Build history of the part. All positions in model axes, mm. A direction names the side the tool comes from. Round coordinates to 2 decimals unless told otherwise and drop trailing zeros. Write each loop counter-clockwise with the first axis right and the second up, starting at its lowest first coordinate (ties: lowest second). Pieces come first, ordered by that corner, then holes.
Item 1: Drop flat-ended pins along their axis: pin 1 Ø4 at (y, z) = (-15, 22.5) entering from +X; pin 2 Ø5 at (y, z) = (-10.5, 54.5) entering from +X; pin 3 Ø2 at (x, y) = (33, -47) entering from -Z. Give the stop position or say it passes through.
Item 2: Band-saw the part on D-D, the plane z = 53. Write the cut outline in (x, y), then the cut area to 3 significant figures.
Item 3: Wall check: probe 1 along Y at (x, z) = (15, 14.5); probe 2 along X at (y, z) = (-12.5, 56); probe 3 along X at (y, z) = (33, 22). Give the ranges that are in metal, low to high.
Item 4: Mould opens along Y. For faces 1 (the flat face through (0, 75, 0)), 2 (the flat face through (-53, 1, 97)), 3 (the flat face through (-18, 77, 38)) say: +Y half, -Y half, draft (parallel to the pull), parting line (faces both ways), or undercut.
Item 5: 3-axis set-ups, long thin cutter, end or side, ignore diameter. For faces 4 (the flat face through (19.75, -1.04, 49.18)), 5 (the flat face through (22.52, -1.08, 50.7)): which of +Z, -Z, +X, -X, +Y, -Y reach the whole face in a straight line?
Item 6: Band-saw the part on C-C, the plane x = -63.5. Write the cut outline in (y, z).
Item 7: Band-saw the part on B-B, the plane y = -11. Write the cut outline in (x, z), then the cut area to 3 significant figures.
Item 8: Band-saw the part on A-A, the plane z = 37. Write the cut outline in (x, y), then the cut area to 3 significant figures.
```python
from build123d import *

# Parameters (mm, degrees)
ESQUISSE1_W             = 154
ESQUISSE1_H             = 154
BOSS_EXTRU_1_DEPTH      = 100
ENL_V_MAT_EXTRU_1_DEPTH = 200.110522073
COQUE2_T                = -3


with BuildPart() as part:
    # Esquisse1 → Boss.-Extru.1 (new body)
    with BuildSketch(Plane.XY):
        Rectangle(ESQUISSE1_W, ESQUISSE1_H)
    extrude(amount=BOSS_EXTRU_1_DEPTH)

    # Esquisse2 → Enlèv. mat.-Extru.1 (cut, through all)
    with BuildSketch(Plane.XZ.offset(77)):
        Polygon((-30.458383107, 100), (77, 0), (77, 100), align=None)
    extrude(amount=-ENL_V_MAT_EXTRU_1_DEPTH, mode=Mode.SUBTRACT)

    # Coque2
    coque2_openings = [part.faces().sort_by_distance(p)[0] for p in [
        (0, 0, 0),
    ]]
    offset(amount=COQUE2_T, openings=coque2_openings, kind=Kind.INTERSECTION)


solid = part.part
```
Results:
1. pin 1: stops at x = 54.97
1. pin 2: stops at x = 21.12
1. pin 3: stops at z = 35.92
2. outline: (-77, -77) - (20.05, -77) - (20.05, 77) - (-77, 77) - close; hole (-74, -74) - (15.64, -74) - (15.64, 74) - (-74, 74) - close
2. area: 1,680 mm2
3. probe 1: y = -77 to -74, 74 to 77
3. probe 2: x = -77 to -74, 12.42 to 16.82
3. probe 3: x = -77 to -74, 48.96 to 53.36
4. face 1: draft
4. face 2: undercut
4. face 3: +Y half
5. face 4: -Z
5. face 5: +Z, +X, +Y, -Y
6. outline: (-77, 0) - (-74, 0) - (-74, 97) - (74, 97) - (74, 0) - (77, 0) - (77, 100) - (-77, 100) - close
7. outline: (-77, 0) - (-74, 0) - (-74, 97) - (-31.64, 97) - (72.6, 0) - (77, 0) - (-30.46, 100) - (-77, 100) - close
7. area: 863 mm2
8. outline: (-77, -77) - (37.24, -77) - (37.24, 77) - (-77, 77) - close; hole (-74, -74) - (32.84, -74) - (32.84, 74) - (-74, 74) - close
8. area: 1,780 mm2
